Check sheet for the modelled part. Datum: model origin and axes. Units: mm. A direction names the side the tool comes from. Round coordinates to 2 decimals unless told otherwise and drop trailing zeros. Write each loop counter-clockwise with the first axis right and the second up, starting at its lowest first coordinate (ties: lowest second). Pieces come first, ordered by that corner, then holes. Notation, with made-up numbers: (87.25, -8.5) -> (126.25, -8.5) arc R30 cw to (126.25, 25.5) -> close; hole circle Ø9 at (52.25, 78.25). An arc over 180 degrees is marked (long way). One line per item, written item: value.
from build123d import *

# Parameters (mm, degrees)
EXTRUDE_1_DEPTH          = 149
SKETCH_7_R               = 3.25
CUT_EXTRUDE_3_DEPTH      = 1.3
SKETCH_8_R               = 1.75
CUT_EXTRUDE_4_DEPTH      = 166.14263547
PATTERN_CIRCULAR_1_COUNT = 3
PATTERN_CIRCULAR_1_ANGLE = 40
SKETCH_9_R               = 3.25
CUT_EXTRUDE_5_DEPTH      = 1.3
SKETCH_10_R              = 1.75
CUT_EXTRUDE_6_DEPTH      = 166.14263547
PATTERN_CIRCULAR_2_COUNT = 5
PATTERN_CIRCULAR_2_ANGLE = 80


with BuildPart() as part:
    # Эскиз1 → Бобышка-Вытянуть1 (new body)
    with BuildSketch(Plane(origin=(0, 0, 0), x_dir=(1, 0, 0), z_dir=(0, 1, 0))):
        with BuildLine():
            Line((-47.135590279, -12.793597189), (-48.562738521, -6.531495034))
            ThreePointArc((-48.562738521, -6.531495034), (-46.263287314, 16.146462365), (-33.952444786, 35.330319742))
            Line((-33.952444786, 35.330319742), (-27.047555214, 40.858655839))
            ThreePointArc((-27.047555214, 40.858655839), (-25.453757982, 41.870111113), (-23.822185811, 42.819428571))
            ThreePointArc((-23.822185811, 42.819428571), (-14.231160733, 46.887888246), (-3.996798719, 48.836723887))
            Line((-3.996798719, 48.836723887), (-3.996798719, 49.84))
            ThreePointArc((-3.996798719, 49.84), (-2, 49.959983987), (0, 50))
            Line((0, 50), (0, 51))
            ThreePointArc((0, 51), (-39.236846594, 32.580206711), (-50.131159715, -9.373730613))
            Line((-50.131159715, -9.373730613), (-49.096909721, -9.138022536))
            Line((-49.096909721, -9.138022536), (-48.208090279, -13.038022536))
            Line((-48.208090279, -13.038022536), (-47.135590279, -12.793597189))
        make_face()
    extrude(amount=EXTRUDE_1_DEPTH)

    # Эскиз7 → Вырез-Вытянуть3 (cut)
    with BuildSketch(Plane.ZY.offset(51)):
        with Locations((0, 4)):
            Circle(SKETCH_7_R)
    cut_extrude_3 = extrude(amount=-CUT_EXTRUDE_3_DEPTH, mode=Mode.SUBTRACT)

    # Эскиз8 → Вырез-Вытянуть4 (cut, through all)
    with BuildSketch(Plane.ZY.offset(49.7)):
        with Locations((0, 4)):
            Circle(SKETCH_8_R)
    cut_extrude_4 = extrude(amount=-CUT_EXTRUDE_4_DEPTH, mode=Mode.SUBTRACT)

    # Круговой массив1: Вырез-Вытянуть3, Вырез-Вытянуть4 ×3 about axis, 1 skipped
    pattern_circular_1_axis = Axis((0, 0, 0), (0, -1, 0))
    add([cut_extrude_3.rotate(pattern_circular_1_axis, i * PATTERN_CIRCULAR_1_ANGLE / (PATTERN_CIRCULAR_1_COUNT - 1)) for i in range(1, PATTERN_CIRCULAR_1_COUNT) if i not in (1,)], mode=Mode.SUBTRACT)
    add([cut_extrude_4.rotate(pattern_circular_1_axis, i * PATTERN_CIRCULAR_1_ANGLE / (PATTERN_CIRCULAR_1_COUNT - 1)) for i in range(1, PATTERN_CIRCULAR_1_COUNT) if i not in (1,)], mode=Mode.SUBTRACT)

    # Эскиз9 → Вырез-Вытянуть5 (cut)
    with BuildSketch(Plane.ZY.offset(51)):
        with Locations((0, 145)):
            Circle(SKETCH_9_R)
    cut_extrude_5 = extrude(amount=-CUT_EXTRUDE_5_DEPTH, mode=Mode.SUBTRACT)

    # Эскиз10 → Вырез-Вытянуть6 (cut, through all)
    with BuildSketch(Plane.ZY.offset(49.7)):
        with Locations((0, 145)):
            Circle(SKETCH_10_R)
    cut_extrude_6 = extrude(amount=-CUT_EXTRUDE_6_DEPTH, mode=Mode.SUBTRACT)

    # Круговой массив2: Вырез-Вытянуть5, Вырез-Вытянуть6 ×5 about axis, 2 skipped
    pattern_circular_2_axis = Axis((0, 149, 0), (0, -1, 0))
    add([cut_extrude_5.rotate(pattern_circular_2_axis, i * PATTERN_CIRCULAR_2_ANGLE / (PATTERN_CIRCULAR_2_COUNT - 1)) for i in range(1, PATTERN_CIRCULAR_2_COUNT) if i not in (1, 3)], mode=Mode.SUBTRACT)
    add([cut_extrude_6.rotate(pattern_circular_2_axis, i * PATTERN_CIRCULAR_2_ANGLE / (PATTERN_CIRCULAR_2_COUNT - 1)) for i in range(1, PATTERN_CIRCULAR_2_COUNT) if i not in (1, 3)], mode=Mode.SUBTRACT)


solid = part.part
Item 1: Sectioned sample at C-C on y = 76. Enter the section's corners in (x, z).
Answer:
outline: (-50.13, 9.37) arc R51 ccw to (0, -51) -> (0, -50) arc R50 cw to (-4, -49.84) -> (-4, -48.84) arc R49 cw to (-27.05, -40.86) -> (-33.95, -35.33) arc R49 cw to (-48.56, 6.53) -> (-47.14, 12.79) -> (-48.21, 13.04) -> (-49.1, 9.14) -> close
Item 2: Sectioned sample at D-D on x = -16. Enter the section's corners in (y, z).
Answer:
outline: (0, -48.43) -> (149, -48.43) -> (149, -46.31) -> (0, -46.31) -> close
Item 3: Mould release check, pull along X, two halves, no side actions. Record for faces 1 (the cylindrical face through (-46.37, 73.46, -15.84)), 2 (the flat face through (-39, 149, -31)), 3 (the cylindrical face through (-38.305, 148.222, -32.694)): pulls with the +X half, pulls with the -X half, needs draft (parallel to the pull), parting line crosses it, or undercut.
Answer:
face 1: pulls with the +X half
face 2: needs draft
face 3: undercut
Item 4: Tool access check on faces 4 (the flat face through (-39, 0, -31)), 5 (the cylindrical face through (-49.34, 146.18, -1.29)), 6 (the flat face through (-38.972, 2.601, -30.875)), 7 (the cylindrical face through (-50.359, 7.222, -0.423)), 8 (the flat face through (-47.84, 73.46, 9.71)). Record the directions out of +Z, -Z, +X, -X, +Y, -Y that give a thin tool (end or side, any length) a straight path to the whole face; none if there is none.
Answer:
face 4: +Z, -Z, +X, -X, -Y
face 5: +X, -X
face 6: none
face 7: -X
face 8: +X, +Y, -Y
Item 5: Sectioned sample at B-B on y = 4. Enter the section's corners in (x, z).
Answer:
outline: (-50.9, -3.25) arc R51 ccw to (-41.08, -30.23) -> (-40.16, -29.46) -> (-39.2, -30.61) -> (-38.64, -30.14) arc R49 cw to (-48.97, -1.75) -> (-49.7, -1.75) -> (-49.7, -3.25) -> close; (-50.9, 3.25) -> (-49.7, 3.25) -> (-49.7, 1.75) -> (-48.97, 1.75) arc R49 cw to (-48.56, 6.53) -> (-47.14, 12.79) -> (-48.21, 13.04) -> (-49.1, 9.14) -> (-50.13, 9.37) arc R51 ccw to start; (-36.95, -33.29) -> (-35.98, -34.44) -> (-36.9, -35.21) arc R51 ccw to (0, -51) -> (0, -50) arc R50 cw to (-4, -49.84) -> (-4, -48.84) arc R49 cw to (-27.05, -40.86) -> (-33.95, -35.33) arc R49 cw to (-36.39, -32.82) -> close
Item 6: Thickness scan on line 1 (Y direction, x = -50, z = 0); line 2 (X direction, y = 66, z = 1); line 3 (Z direction, x = -40, y = 95). Record the ranges inside material, lowest first.
Answer:
line 1: y = 0 to 0.75, 7.25 to 141.75, 148.25 to 149
line 2: x = -50.99 to -48.99
line 3: z = -31.64 to -28.3
Item 7: Depth check by flat-ended pin: P1, Ø12, axis at x = -28.5, y = 55.5, coming from the -Z side; P2, Ø0.8, axis at y = 61.5, z = -49, coming from the +X side; P3, Ø6, axis at x = -11, y = 47.5, coming from the +Z side. Enter the tip coordinate at first touch or a pass-through.
Answer:
P1: stops at z = -45.77
P2: stops at x = -4
P3: stops at z = -46.96
Item 8: Sectioned sample at A-A on z = 0. Enter the section's corners in (x, y).
Answer:
outline: (-51, 0) -> (-49, 0) -> (-49, 2.25) -> (-49.7, 2.25) -> (-49.7, 0.75) -> (-51, 0.75) -> close; (-51, 7.25) -> (-49.7, 7.25) -> (-49.7, 5.75) -> (-49, 5.75) -> (-49, 143.25) -> (-49.7, 143.25) -> (-49.7, 141.75) -> (-51, 141.75) -> close; (-51, 148.25) -> (-49.7, 148.25) -> (-49.7, 146.75) -> (-49, 146.75) -> (-49, 149) -> (-51, 149) -> close
